Here's the drawing with two shaded views (mm, measured from the low corner). I have some questions. A direction names the side the tool comes from. Round coordinates to 2 decimals unless told otherwise and drop trailing zeros. Loops run counter-clockwise (first coordinate to the right, second up) from the corner with the lowest first, then second, coordinate; pieces in that order, holes last. Notation, with made-up numbers: M -6.5,-11 L 4.5,-11 A25 cw 4.5,20 Z; hole C 4,85 d2. An arc over 180 degrees is marked long. One line per item, written item: value. Start each with the question number.
Q1. Thinking about a two-plate mould opening in Y: for the marked faces 1, 2 and 3, which applies, released by +Y, released by -Y, zero draft, split by the parting line, or undercut?
Q2. Please list where these lines run through material, in increasing order: line 1 along Y through (x, z) = (8, 4.75); line 2 along X through (y, z) = (4.75, 10.25) (1 decimal); line 3 along Y through (x, z) = (9.5, 2.25) (1 decimal).
Q3. I'm going to push flat-ended pins straight in: pin 1 Ø5 at (x, z) = (9.5, 4.5) entering from +Y; pin 2 Ø4 at (x, y) = (11, 7) entering from +Z (1 decimal); pin 3 Ø2 at (x, y) = (7, 10) entering from +Z; pin 4 Ø5 at (y, z) = (5, 4.5) entering from -X. Where does each tip first touch, or does it pass through?
Q4. Imagine slicing it at B-B (z = 11.25). Please give me the cut outline in (x, y) (1 decimal).
Q5. Imagine slicing it at A-A (z = 5.75). Please give me the cut outline in (x, y) (1 decimal).
Q6. Which directions (+Z, -Z, +X, -X, +Y, -Y) give clear straight access to the entire face, cutting with the end or side of a thin tool? Please do the marked faces 4 and 5.
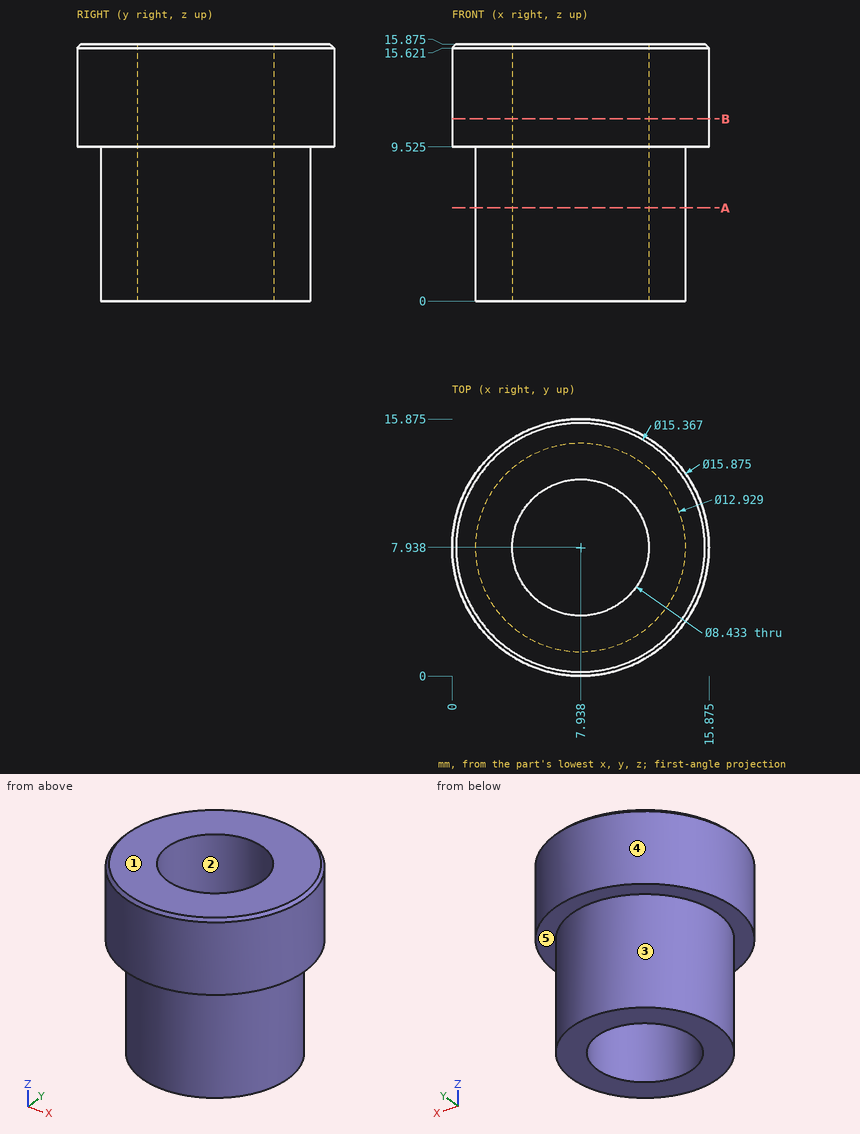
Report:
1. face 1: zero draft
1. face 2: undercut
1. face 3: split by the parting line
2. line 1: y = 1.47 to 3.72, 12.15 to 14.4
2. line 2: x = 0.7 to 5.2, 10.7 to 15.2
2. line 3: y = 1.7 to 4, 11.9 to 14.2
3. pin 1: stops at y = 14.4
3. pin 2: stops at z = 15.9
3. pin 3: passes through
3. pin 4: stops at x = 1.49
4. outline: C 7.9,7.9 d15.9; hole C 7.9,7.9 d8.4
5. outline: C 7.9,7.9 d12.9; hole C 7.9,7.9 d8.4
6. face 4: +Z, -Z
6. face 5: -Z
